```python
from build123d import *

# Parameters (mm, degrees)
F0_W           = 100
F0_H           = 120
F1_DEPTH       = 13
F3_D           = 6.6
F4_D           = 6.6
F4_CBORE_D     = 11.25
F4_CBORE_DEPTH = 6
F5_R           = 8


with BuildPart() as f1:
    # F0 (on Front) → F1 (new body)
    with BuildSketch(Plane.XZ):
        with Locations((50, 60)):
            Rectangle(F0_W, F0_H)
    extrude(amount=F1_DEPTH)

    # F3 (through all)
    with Locations(Plane.XZ.offset(13)):
        with Locations((80, 30), (20, 40)):
            Hole(F3_D / 2)

    # F4 (through all)
    with Locations(Plane.XZ.offset(13)):
        with Locations((50, 70), (50, 45)):
            CounterBoreHole(F4_D / 2, F4_CBORE_D / 2, F4_CBORE_DEPTH)

    # F5
    f5_edges = [f1.edges().sort_by_distance(p)[0] for p in [
        (100, -6.5, 120),
        (100, -6.5, 0),
        (0, -6.5, 120),
        (0, -6.5, 0),
    ]]
    fillet(f5_edges, radius=F5_R)


solid = f1.part
```
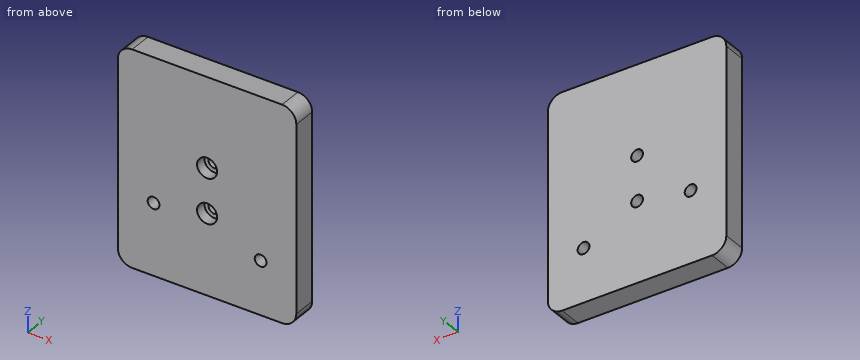
Here's how the part is built. I have some questions about the finished solid (model axes, mm). Give positions to 0.01 mm unless a question says otherwise; leave off trailing zeros. Order: outer loops, then holes, each group sorted by start corner. A loop starts at its lowest first (then second) coordinate and runs counter-clockwise, first axis right, second up. Notation, with made-up numbers: M 30.25,10.5 L 50.25,10.5 A26 cw 50.25,26.5 Z; hole C 31.5,-19.5 d5. An arc over 180 degrees is marked long. Use a Markdown table: item, result. Add a question column.
1. I need wall thicknesses on probe 1 along Z at (x, y) = (50, -9.15) (3 decimals); probe 2 along Z at (x, y) = (50, -3.5); probe 3 along Z at (x, y) = (20, -3.75). Which ranges of each line are inside material? Lowest first, please. Write a range as from..to.
2. Suppose I cut it at C-C (y = -4.5). List the corners of the cut face in (x, z) for me.
3. Suppose I cut it at A-A (z = 30). List the corners of the cut face in (x, y) for me, and give its area (3 significant figures).
4. For pin 1 Ø9 at (x, z) = (50, 70) entering from -Y, with a flat end and sliding along its axis, tell me the tip position at first contact or that it passes through.
5. Suppose I cut it at D-D (x = 49.5). List the corners of the cut face in (y, z) for me, and give its area (3 significant figures).
6. Suppose I cut it at B-B (x = 80). List the corners of the cut face in (y, z) for me.
Results list:
| question | item | result |
|---|---|---|
| 1 | probe 1 | z = 0..39.375, 50.625..64.375, 75.625..120 |
| 1 | probe 2 | z = 0..41.7, 48.3..66.7, 73.3..120 |
| 1 | probe 3 | z = 0..36.7, 43.3..120 |
| 2 | outline | M 0,8 A8 ccw 8,0 L 92,0 A8 ccw 100,8 L 100,112 A8 ccw 92,120 L 8,120 A8 ccw 0,112 Z; hole C 20,40 d6.6; hole C 50,45 d6.6; hole C 50,70 d6.6; hole C 80,30 d6.6 |
| 3 | outline | M 0,-13 L 76.7,-13 L 76.7,0 L 0,0 Z; M 83.3,-13 L 100,-13 L 100,0 L 83.3,0 Z |
| 3 | area | 1,210 mm² |
| 4 | pin 1 | stops at y = -7 |
| 5 | outline | M -13,0 L 0,0 L 0,41.74 L -7,41.74 L -7,39.4 L -13,39.4 Z; M -13,50.6 L -7,50.6 L -7,48.26 L 0,48.26 L 0,66.74 L -7,66.74 L -7,64.4 L -13,64.4 Z; M -13,75.6 L -7,75.6 L -7,73.26 L 0,73.26 L 0,120 L -13,120 Z |
| 5 | area | 1,330 mm² |
| 6 | outline | M -13,0 L 0,0 L 0,26.7 L -13,26.7 Z; M -13,33.3 L 0,33.3 L 0,120 L -13,120 Z |
